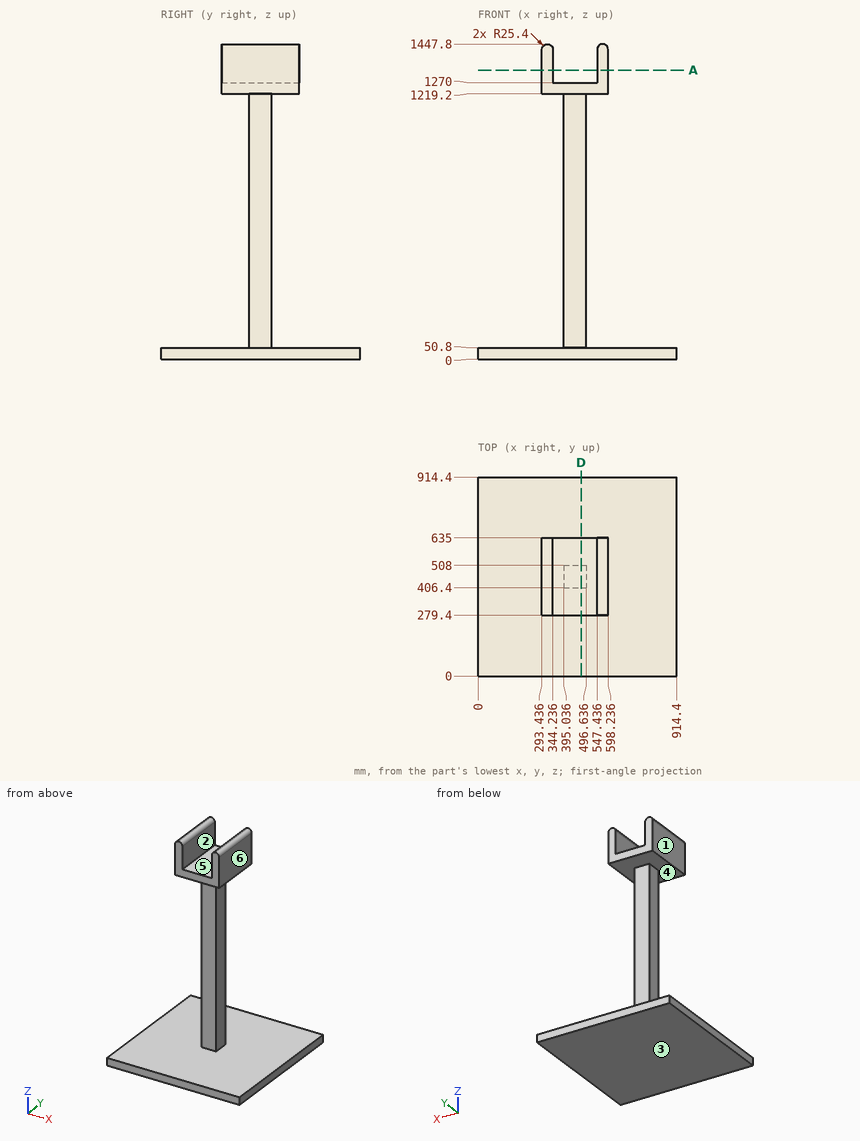
Study the drawing (mm; zero at the part's minimum x, y, z) and answer. A direction names the side the tool comes from. Give positions to 0.01 mm unless a question says otherwise; leave off trailing zeros. Order: outer loops, then holes, each group sorted by start corner. A loop starts at its lowest first (then second) coordinate and runs counter-clockwise, first axis right, second up. Notation, with made-up numbers: (68.5, 75) - (104.5, 75) arc R15 ccw to (104.5, 104) - close; hole circle Ø1 at (71.25, -22.5). An arc over 180 degrees is marked (long way). Answer in a Markdown table with one row per item. Add a question column.
Q1. Given P1, Ø8, axis at x = 402.5, y = 564.5, coming from the +Z side; P2, Ø10, axis at x = 616, y = 347, coming from the +Z side; P3, Ø6, axis at x = 719, y = 771.5, coming from the -Z side, each flat-ended and moving along its own axis, determine where each tip first touches the part or whether it passes through.
Q2. Find the intervals of material crossed by line 1 along Y through (x, z) = (400, 623); line 2 along Z through (x, y) = (404.5, 390); line 3 along Z through (x, y) = (216.5, 810.5), in increasing order. Write a range as [from, to].
Q3. The part is cut by section D-D (x = 474). Determine the outline of the cut face in (y, z), then the cut area to 3 significant figures.
Q4. For a pull along X with two mould halves and no side action, classify the marked faces 4, 5 and 6 as released by +X, released by -X, zero draft, split by the parting line, or undercut.
Q5. Which of the six approach directions +Z, -Z, +X, -X, +Y, -Y give full straight-line access (tool end or side, diameter ignored) to the marked faces 1, 2 and 3?
Q6. The part is cut by section A-A (z = 1328). Determine the outline of the cut face in (x, y).
Determined:
| question | item | result |
|---|---|---|
| 1 | P1 | stops at z = 1270 |
| 1 | P2 | stops at z = 50.8 |
| 1 | P3 | stops at z = 0 |
| 2 | line 1 | y = [406.4, 508] |
| 2 | line 2 | z = [0, 50.8], [1219.2, 1270] |
| 2 | line 3 | z = [0, 50.8] |
| 3 | outline | (0, 0) - (914.4, 0) - (914.4, 50.8) - (508, 50.8) - (508, 1219.2) - (635, 1219.2) - (635, 1270) - (279.4, 1270) - (279.4, 1219.2) - (406.4, 1219.2) - (406.4, 50.8) - (0, 50.8) - close |
| 3 | area | 183,000 mm² |
| 4 | face 4 | zero draft |
| 4 | face 5 | undercut |
| 4 | face 6 | released by +X |
| 5 | face 1 | +Z, -X, +Y, -Y |
| 5 | face 2 | +Z, +Y, -Y |
| 5 | face 3 | -Z, +X, -X, +Y, -Y |
| 6 | outline | (293.44, 279.4) - (344.24, 279.4) - (344.24, 635) - (293.44, 635) - close; (547.44, 279.4) - (598.24, 279.4) - (598.24, 635) - (547.44, 635) - close |
